```python
from build123d import *

# Parameters (mm, degrees)
SKETCH1_W           = 590
SKETCH1_H           = 609.3
BOSS_EXTRUDE1_DEPTH = 10
SKETCH2_R           = 50
CUT_EXTRUDE3_DEPTH  = 425.189371036
SKETCH3_W           = 400
SKETCH3_H           = 400
BOSS_EXTRUDE6_DEPTH = 10


with BuildPart() as part:
    # Sketch1 → Boss-Extrude1 (new body)
    with BuildSketch(Plane(origin=(0, 0, 0), x_dir=(1, 0, 0), z_dir=(0, 1, 0))):
        Rectangle(SKETCH1_W, SKETCH1_H)
    extrude(amount=BOSS_EXTRUDE1_DEPTH)

    # Sketch2 → Cut-Extrude3 (cut, through all)
    with BuildSketch(Plane(origin=(0, 10, 0), x_dir=(1, 0, 0), z_dir=(0, 1, 0))):
        with Locations(Location((0, -234.65, 0), (0, 0, 270))):
            Circle(SKETCH2_R)
    extrude(amount=-CUT_EXTRUDE3_DEPTH, mode=Mode.SUBTRACT)

    # Sketch3 → Boss-Extrude6 (add)
    with BuildSketch(Plane(origin=(0, 10, -62.246477908), x_dir=(1, 0, 0), z_dir=(0, 1, 0))):
        with Locations((0, -0.096477908)):
            Rectangle(SKETCH3_W, SKETCH3_H)
    extrude(amount=BOSS_EXTRUDE6_DEPTH)


solid = part.part
```
The model under review builds one solid part; all positions refer to its coordinate system, in mm. Give positions to 0.01 mm unless a question says otherwise; leave off trailing zeros. Loops run counter-clockwise (first coordinate to the right, second up) from the corner with the lowest first, then second, coordinate; pieces in that order, holes last. Notation, with made-up numbers: (-0.5, 46.5) - (23.5, 46.5) arc R26 cw to (23.5, 83.5) - close; hole circle Ø2 at (74.25, -30.75). An arc over 180 degrees is marked (long way). Answer as a JSON object with one key per item and string values.
Q1. Insertion check: pin 1 (8 mm diameter, centred on x = -21.5, y = 15, fed in from -Z); pin 2 (2 mm diameter, centred on x = -200.5, z = -136, fed in from -Y); pin 3 (5 mm diameter, centred on x = 40, y = 17, fed in from +Z); pin 4 (1 mm diameter, centred on x = -183, z = 183, fed in from +Y). Each pin has a flat end and moves straight along its axis. Give the tip position at first contact, or say it passes through.
Worked out:
{"pin 1": "stops at z = -262.15", "pin 2": "stops at y = 0", "pin 3": "stops at z = 137.85", "pin 4": "stops at y = 10"}
Q2. To check wall thickness, follow line 1 along X through (y, z) = (5.5, 234.65); line 2 along Y through (x, z) = (238.5, 246.5); line 3 along X through (y, z) = (13.75, -254.5). State the ranges of each line that lie inside material, in increasing order.
Worked out:
{"line 1": "x = -295 to -50, 50 to 295", "line 2": "y = 0 to 10", "line 3": "x = -200 to 200"}
Q3. Mouldability with a two-part tool opening along Z and no side actions: class faces 1 (the cylindrical face through (15.02, 5.07, 282.34)), 2 (the flat face through (-3, 20, -65)) as +Z half, -Z half, draft (parallel to the pull), parting line (faces both ways), or undercut.
Worked out:
{"face 1": "undercut", "face 2": "draft"}
Q4. Add section B-B on z = 234.65. State the section outline as (x, y) points, plus the area to 3 significant figures.
Worked out:
{"outline": "(-295, 0) - (-50, 0) - (-50, 10) - (-295, 10) - close; (50, 0) - (295, 0) - (295, 10) - (50, 10) - close", "area": "4,900 mm^2"}
Q5. Add section A-A on x = 0. State the section outline as (y, z) points.
Worked out:
{"outline": "(0, -304.65) - (10, -304.65) - (10, -262.15) - (20, -262.15) - (20, 137.85) - (10, 137.85) - (10, 184.65) - (0, 184.65) - close; (0, 284.65) - (10, 284.65) - (10, 304.65) - (0, 304.65) - close"}
Q6. Add section C-C on z = -57.5. State the section outline as (x, y) points, plus the area to 3 significant figures.
Worked out:
{"outline": "(-295, 0) - (295, 0) - (295, 10) - (200, 10) - (200, 20) - (-200, 20) - (-200, 10) - (-295, 10) - close", "area": "9,900 mm^2"}
Q7. Add section D-D on x = 79. State the section outline as (y, z) points.
Worked out:
{"outline": "(0, -304.65) - (10, -304.65) - (10, -262.15) - (20, -262.15) - (20, 137.85) - (10, 137.85) - (10, 304.65) - (0, 304.65) - close"}
